Can you work these out from the model? Positions are in its coordinate system, mm. Round coordinates to 2 decimals unless told otherwise and drop trailing zeros. Write each loop counter-clockwise with the first axis right and the second up, starting at its lowest first coordinate (ties: lowest second). Pieces come first, ordered by that corner, then holes. Notation, with made-up numbers: M 67.25,59 L 109.25,59 A22 cw 109.25,81 Z; hole C 70,43.25 d8. An arc over 180 degrees is marked long. Use one line per item in the form item = value. Start each with the question number.
```python
from build123d import *

# Parameters (mm, degrees)
F0_W     = 152.4
F0_H     = 914.4
F0_R     = 7.9375
F1_DEPTH = 12.7


with BuildPart() as f1:
    # F0 (on Top) → F1 (new body)
    with BuildSketch(Plane.XY):
        with Locations((50.8, 457.2)):
            Rectangle(F0_W, F0_H)
        with Locations((0, 50.8)):
            Circle(F0_R, mode=Mode.SUBTRACT)
        with Locations((0, 101.6)):
            Circle(F0_R, mode=Mode.SUBTRACT)
        with Locations((0, 152.4)):
            Circle(F0_R, mode=Mode.SUBTRACT)
        with Locations((0, 203.2)):
            Circle(F0_R, mode=Mode.SUBTRACT)
        with Locations((50.8, 50.8)):
            Circle(F0_R, mode=Mode.SUBTRACT)
        with Locations((50.8, 101.6)):
            Circle(F0_R, mode=Mode.SUBTRACT)
        with Locations((50.8, 152.4)):
            Circle(F0_R, mode=Mode.SUBTRACT)
        with Locations((50.8, 203.2)):
            Circle(F0_R, mode=Mode.SUBTRACT)
        with Locations((0, 254)):
            Circle(F0_R, mode=Mode.SUBTRACT)
        with Locations((0, 304.8)):
            Circle(F0_R, mode=Mode.SUBTRACT)
        with Locations((0, 355.6)):
            Circle(F0_R, mode=Mode.SUBTRACT)
        with Locations((0, 406.4)):
            Circle(F0_R, mode=Mode.SUBTRACT)
        with Locations((50.8, 254)):
            Circle(F0_R, mode=Mode.SUBTRACT)
        with Locations((50.8, 304.8)):
            Circle(F0_R, mode=Mode.SUBTRACT)
        with Locations((50.8, 355.6)):
            Circle(F0_R, mode=Mode.SUBTRACT)
        with Locations((50.8, 406.4)):
            Circle(F0_R, mode=Mode.SUBTRACT)
        with Locations((101.6, 50.8)):
            Circle(F0_R, mode=Mode.SUBTRACT)
        with Locations((101.6, 101.6)):
            Circle(F0_R, mode=Mode.SUBTRACT)
        with Locations((101.6, 152.4)):
            Circle(F0_R, mode=Mode.SUBTRACT)
        with Locations((101.6, 203.2)):
            Circle(F0_R, mode=Mode.SUBTRACT)
        with Locations((101.6, 254)):
            Circle(F0_R, mode=Mode.SUBTRACT)
        with Locations((101.6, 304.8)):
            Circle(F0_R, mode=Mode.SUBTRACT)
        with Locations((101.6, 355.6)):
            Circle(F0_R, mode=Mode.SUBTRACT)
        with Locations((101.6, 406.4)):
            Circle(F0_R, mode=Mode.SUBTRACT)
        with Locations((0, 457.2)):
            Circle(F0_R, mode=Mode.SUBTRACT)
        with Locations((0, 508)):
            Circle(F0_R, mode=Mode.SUBTRACT)
        with Locations((0, 558.8)):
            Circle(F0_R, mode=Mode.SUBTRACT)
        with Locations((0, 609.6)):
            Circle(F0_R, mode=Mode.SUBTRACT)
        with Locations((0, 660.4)):
            Circle(F0_R, mode=Mode.SUBTRACT)
        with Locations((50.8, 457.2)):
            Circle(F0_R, mode=Mode.SUBTRACT)
        with Locations((50.8, 508)):
            Circle(F0_R, mode=Mode.SUBTRACT)
        with Locations((50.8, 558.8)):
            Circle(F0_R, mode=Mode.SUBTRACT)
        with Locations((50.8, 609.6)):
            Circle(F0_R, mode=Mode.SUBTRACT)
        with Locations((50.8, 660.4)):
            Circle(F0_R, mode=Mode.SUBTRACT)
        with Locations((0, 711.2)):
            Circle(F0_R, mode=Mode.SUBTRACT)
        with Locations((0, 762)):
            Circle(F0_R, mode=Mode.SUBTRACT)
        with Locations((0, 812.8)):
            Circle(F0_R, mode=Mode.SUBTRACT)
        with Locations((0, 863.6)):
            Circle(F0_R, mode=Mode.SUBTRACT)
        with Locations((50.8, 711.2)):
            Circle(F0_R, mode=Mode.SUBTRACT)
        with Locations((50.8, 762)):
            Circle(F0_R, mode=Mode.SUBTRACT)
        with Locations((50.8, 812.8)):
            Circle(F0_R, mode=Mode.SUBTRACT)
        with Locations((50.8, 863.6)):
            Circle(F0_R, mode=Mode.SUBTRACT)
        with Locations((101.6, 457.2)):
            Circle(F0_R, mode=Mode.SUBTRACT)
        with Locations((101.6, 508)):
            Circle(F0_R, mode=Mode.SUBTRACT)
        with Locations((101.6, 558.8)):
            Circle(F0_R, mode=Mode.SUBTRACT)
        with Locations((101.6, 609.6)):
            Circle(F0_R, mode=Mode.SUBTRACT)
        with Locations((101.6, 660.4)):
            Circle(F0_R, mode=Mode.SUBTRACT)
        with Locations((101.6, 711.2)):
            Circle(F0_R, mode=Mode.SUBTRACT)
        with Locations((101.6, 762)):
            Circle(F0_R, mode=Mode.SUBTRACT)
        with Locations((101.6, 812.8)):
            Circle(F0_R, mode=Mode.SUBTRACT)
        with Locations((101.6, 863.6)):
            Circle(F0_R, mode=Mode.SUBTRACT)
    extrude(amount=F1_DEPTH)


solid = f1.part
```
1. Please list where these lines run through material, in increasing order: line 1 along X through (y, z) = (556.5, 5.25); line 2 along X through (y, z) = (251, 2.5).
2. If we mould it in two halves opening along X, with no side actions, what happens to faces 1 (the face through (33, 464, 12.7)), 2 (the face through (44.5, 299.97, 6.26))? For each: pulls with the +X half, pulls with the -X half, needs draft (parallel to the pull), parting line crosses it, or undercut.
3. If we section it at A-A (y = 457.2): List the corners of the cut face in (x, z) for me, and give its area (3 significant figures).
4. If we section it at B-B (x = 50.8): State how many separate pieces and enclosed holes the cut face has, and give its area (3 significant figures).
5. Will these pins go through, and if not, where does the flat tip stop? pin 1 (14.5 mm diameter, centred on x = 0, y = 304.8, fed in from +Z); pin 2 (1 mm diameter, centred on x = 15.5, y = 146, fed in from -Z).
Model answer:
q1.line_1 = -25.4 to -7.6, 7.6 to 43.2, 58.4 to 94, 109.2 to 127
q1.line_2 = -25.4 to -7.35, 7.35 to 43.45, 58.15 to 94.25, 108.95 to 127
q2.face_1 = needs draft
q2.face_2 = undercut
q3.outline = M -25.4,0 L -7.94,0 L -7.94,12.7 L -25.4,12.7 Z; M 7.94,0 L 42.86,0 L 42.86,12.7 L 7.94,12.7 Z; M 58.74,0 L 93.66,0 L 93.66,12.7 L 58.74,12.7 Z; M 109.54,0 L 127,0 L 127,12.7 L 109.54,12.7 Z
q3.area = 1,330 mm2
q4.separate_pieces = 18
q4.enclosed_holes = 0
q4.area = 8,190 mm2
q5.pin_1 = through
q5.pin_2 = 0
